Geometry: final body of the model. Coordinates: model frame, mm. Face numbers are marked on the shaded views. A direction names the side the tool comes from. Round coordinates to 2 decimals unless told otherwise and drop trailing zeros. Write each loop counter-clockwise with the first axis right and the second up, starting at its lowest first coordinate (ties: lowest second). Pieces come first, ordered by that corner, then holes. Notation, with made-up numbers: M 57,-22 L 85,-22 A15 cw 85,-18 Z; hole C 5,24 d2. An arc over 180 degrees is marked long. Answer as CSV lines item,"result". Start each with the question number.
Q1. First-contact query: pin 1 (1 mm diameter, centred on x = 14, z = 9.5, fed in from -Y); pin 2 (12 mm diameter, centred on x = 11.5, z = 35, fed in from -Y); pin 3 (3.5 mm diameter, centred on x = 8.5, y = 1.5, fed in from -Z). Flat tips, straight axial feed; report the tip coordinate or a pass-through.
Q2. Mould query, pull axis Y, two halves, no side actions, for the marked faces 1, 2 and 3. Classes: pulls with the +Y half, pulls with the -Y half, needs draft (parallel to the pull), parting line crosses it, or undercut.
Q3. Ray query, probe 1 along Y at (x, z) = (16.75, 12); probe 2 along Y at (x, z) = (11.75, 13); probe 3 along Y at (x, z) = (17.5, 14.5). Return the intervals inside material, ascending.
Q4. Section query C-C on z = 37.5. Output: boundary loops of the cut face in (x, y).
Q5. Section query B-B on y = 1. Output: boundary loops of the cut face in (x, z), and give its area (3 significant figures).
Q6. Section query A-A on z = 24. Output: boundary loops of the cut face in (x, y), and give its area (3 significant figures).
Q7. Reachability of the marked faces 4, 5 and 6 from +Z, -Z, +X, -X, +Y, -Y: full face, straight path, thin tool, end or side. Return the list, or none.
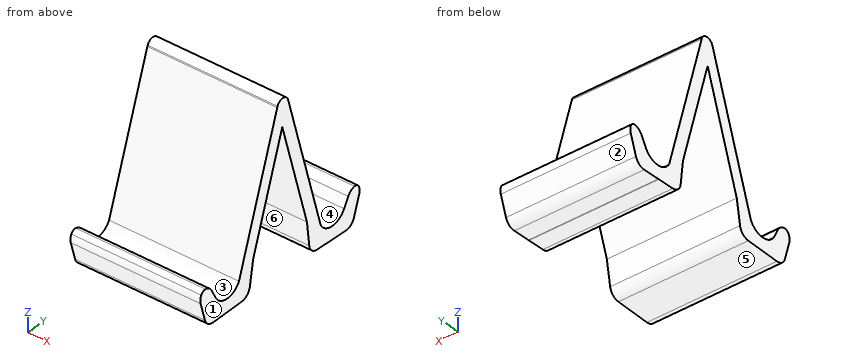
```python
from build123d import *

# Parameters (mm, degrees)
F1_DEPTH    = 25
F2_T1_DEPTH = 35
F2_T3_DEPTH = 33.3163528131
F3_R        = 1
F4_R        = 2


# Not quite as in the source:
# - a fillet or chamfer that OpenCascade refuses, or shapes differently, is made with other operations: its cross-section is extruded or revolved along the edge and cut away or added


with BuildPart() as f1:
    # F0 (on Right) → F1 (new body)
    with BuildSketch(Plane.YZ):
        with BuildLine():
            Line((-6.9323359057, 13.8083724305), (-5, 7.0966093383))
            Line((-5, 7.0966093383), (-0.1434815237, 7.0966093383))
            ThreePointArc((-0.1434815237, 7.0966093383), (-3.0832893136, 7.9619770163), (-5.1434815237, 10.2306636665))
            Line((-5.1434815237, 10.2306636665), (-6.9323359057, 13.8083724305))
        make_face()
        with BuildLine():
            ThreePointArc((-5.1434815237, 10.2306636665), (-3.0832893136, 7.9619770163), (-0.1434815237, 7.0966093383))
            Line((-0.1434815237, 7.0966093383), (0, 7.0966093383))
            ThreePointArc((0, 7.0966093383), (2.9398077898, 7.9619770163), (5, 10.2306636665))
            Line((5, 10.2306636665), (6.0755903162, 13.4044619593))
            Line((6.0755903162, 13.4044619593), (13.0241518458, 33.9079309741))
            Line((13.0241518458, 33.9079309741), (11.8234508953, 38.1539476614))
            Line((11.8234508953, 38.1539476614), (2.6952738362, 11.2189777838))
            ThreePointArc((2.6952738362, 11.2189777838), (-0.1451253509, 9.597004922), (-2.9074135462, 11.3486976553))
            Line((-2.9074135462, 11.3486976553), (-4.6962679282, 14.9264064193))
            Line((-4.6962679282, 14.9264064193), (-6.9323359057, 13.8083724305))
            Line((-6.9323359057, 13.8083724305), (-5.1434815237, 10.2306636665))
        make_face()
        with BuildLine():
            ThreePointArc((5, 10.2306636665), (2.9398077898, 7.9619770163), (0, 7.0966093383))
            Line((0, 7.0966093383), (5, 7.0966093383))
            Line((5, 7.0966093383), (6.0755903162, 13.4044619593))
            Line((6.0755903162, 13.4044619593), (5, 10.2306636665))
        make_face()
        with BuildLine():
            Line((11.8234508953, 38.1539476614), (13.0241518458, 33.9079309741))
            Line((13.0241518458, 33.9079309741), (14.4404213471, 38.0869884254))
            Line((14.4404213471, 38.0869884254), (14.3799488187, 38.3008363155))
            ThreePointArc((14.3799488187, 38.3008363155), (13.1588056017, 39.1706090028), (11.8947803947, 38.3644231928))
            Line((11.8947803947, 38.3644231928), (11.8234508953, 38.1539476614))
        make_face()
        with BuildLine():
            Line((14.4404213471, 38.0869884254), (13.0241518458, 33.9079309741))
            Line((13.0241518458, 33.9079309741), (18.9150818034, 13.075943714))
            Line((18.9150818034, 13.075943714), (19.8269579074, 9.8512930193))
            ThreePointArc((19.8269579074, 9.8512930193), (21.7684346268, 7.4802174812), (24.6601411506, 6.4656414912))
            Line((24.6601411506, 6.4656414912), (24.8034349308, 6.4583039016))
            ThreePointArc((24.8034349308, 6.4583039016), (27.7836505914, 7.1721986247), (29.9571668266, 9.332559297))
            Line((29.9571668266, 9.332559297), (31.9266431601, 12.8141053576))
            Line((31.9266431601, 12.8141053576), (29.7506768723, 14.045028066))
            Line((29.7506768723, 14.045028066), (27.7812005388, 10.5634820055))
            ThreePointArc((27.7812005388, 10.5634820055), (24.9329458702, 8.9553436878), (22.1792103708, 10.7204511366))
            Line((22.1792103708, 10.7204511366), (14.4404213471, 38.0869884254))
        make_face()
        with BuildLine():
            Line((19.8269579074, 9.8512930193), (18.9150818034, 13.075943714))
            Line((18.9150818034, 13.075943714), (19.6666835811, 6.7213395575))
            Line((19.6666835811, 6.7213395575), (24.6601411506, 6.4656414912))
            ThreePointArc((24.6601411506, 6.4656414912), (21.7684346268, 7.4802174812), (19.8269579074, 9.8512930193))
        make_face()
        with BuildLine():
            ThreePointArc((29.9571668266, 9.332559297), (27.7836505914, 7.1721986247), (24.8034349308, 6.4583039016))
            Line((24.8034349308, 6.4583039016), (29.6535987202, 6.2099434249))
            Line((29.6535987202, 6.2099434249), (31.9266431601, 12.8141053576))
            Line((31.9266431601, 12.8141053576), (29.9571668266, 9.332559297))
        make_face()
    extrude(amount=F1_DEPTH)

    # F2: fillet of radius 2 on 4 edges, made by hand

    # F2_s2 → F2_t1 (cut)
    with BuildSketch(Plane.YZ.offset(-5)):
        with BuildLine():
            ThreePointArc((-3.8018407372, 13.1375520373), (-4.9582395872, 14.1404914424), (-6.4851223102, 14.0319792283))
            Line((-6.4851223102, 14.0319792283), (-4.6962679282, 14.9264064193))
            Line((-4.6962679282, 14.9264064193), (-3.8018407372, 13.1375520373))
        make_face()
        with BuildLine():
            ThreePointArc((31.4914499025, 13.0602898993), (29.972114357, 13.2467443186), (28.7659387055, 12.3042550357))
            Line((28.7659387055, 12.3042550357), (29.7506768723, 14.045028066))
            Line((29.7506768723, 14.045028066), (31.4914499025, 13.0602898993))
        make_face()
    extrude(amount=F2_T1_DEPTH, mode=Mode.SUBTRACT)

    # F2_s4 → F2_t3 (cut)
    with BuildSketch(Plane.YZ.offset(-4.1581764065)):
        with BuildLine():
            ThreePointArc((-6.4721671557, 12.2100252573), (-6.3817440303, 13.5668302715), (-5.4446614885, 14.5522096391))
            Line((-5.4446614885, 14.5522096391), (-6.9323359057, 13.8083724305))
            Line((-6.9323359057, 13.8083724305), (-6.4721671557, 12.2100252573))
        make_face()
        with BuildLine():
            ThreePointArc((31.3853376782, 11.2413824514), (31.3644193539, 12.6010363088), (30.4789548914, 13.6330483599))
            Line((30.4789548914, 13.6330483599), (31.9266431601, 12.8141053576))
            Line((31.9266431601, 12.8141053576), (31.3853376782, 11.2413824514))
        make_face()
    extrude(amount=F2_T3_DEPTH, mode=Mode.SUBTRACT)

    # F3
    f3_edges = [f1.edges().sort_by_distance(p)[0] for p in [
        (12.5, -5.926233, 14.214777),
        (12.5, 30.942641, 13.27143),
    ]]
    fillet(f3_edges, radius=F3_R)

    # F4
    f4_edges = [f1.edges().sort_by_distance(p)[0] for p in [
        (12.5, -5, 7.096609),
        (12.5, 5, 7.096609),
        (12.5, 19.666684, 6.72134),
        (12.5, 29.653599, 6.209943),
    ]]
    fillet(f4_edges, radius=F4_R)


solid = f1.part
```
Entries:
1,pin 1,"stops at y = -5.84"
1,pin 2,"stops at y = 8.72"
1,pin 3,"stops at z = 7.1"
2,face 1,"needs draft"
2,face 2,"pulls with the +Y half"
2,face 3,"undercut"
3,probe 1,"y = -6.41 to -3.23, 2.96 to 5.84, 19.04 to 21.82, 28.59 to 31.49"
3,probe 2,"y = -6.54 to -3.73, 3.3 to 6.01, 18.92 to 21.53, 29.42 to 31.13"
3,probe 3,"y = 3.81 to 6.45, 18.51 to 21.11"
4,outline,"M 0,11.6 L 25,11.6 L 25,14.61 L 0,14.61 Z"
5,outline,"M 0,7.1 L 25,7.1 L 25,9.78 L 0,9.78 Z"
5,area,"67.2 mm^2"
6,outline,"M 0,7.03 L 25,7.03 L 25,9.67 L 0,9.67 Z; M 0,15.83 L 25,15.83 L 25,18.42 L 0,18.42 Z"
6,area,"131 mm^2"
7,face 4,"+Z, +X, -X"
7,face 5,"-Z, +X, -X, -Y"
7,face 6,"-Z, +X, -X"
